Part print with two shaded views. Sizes in mm from the minimum x, y, z corner. A direction names the side the tool comes from. Give positions to 0.01 mm unless a question says otherwise; leave off trailing zeros. Write each loop counter-clockwise with the first axis right and the second up, starting at its lowest first coordinate (ties: lowest second). Pieces come first, ordered by that corner, then holes.
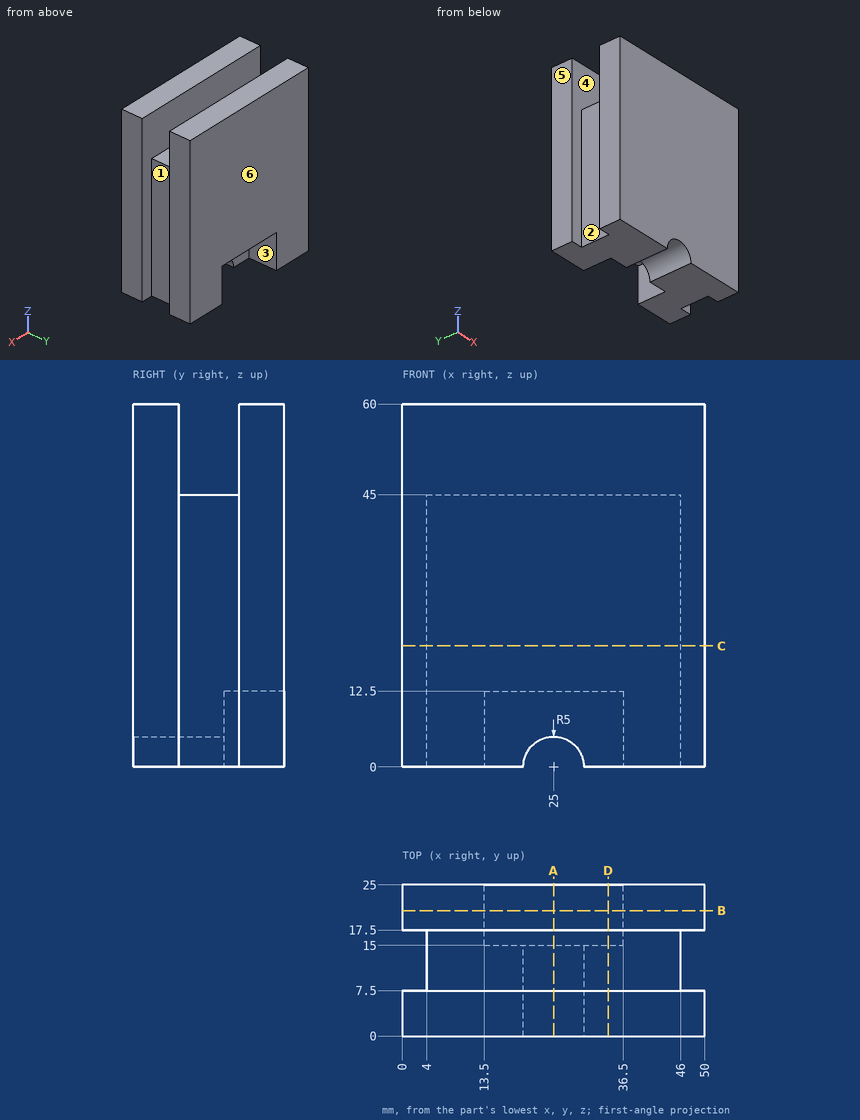
(1) Mould opens along Y. For the marked faces 4, 5 and 6 say: +Y half, -Y half, draft (parallel to the pull), parting line (faces both ways), or undercut.
(2) Saw through at C-C, the plane z = 20. List the corners of the cut face in (x, y).
(3) Saw through at A-A, the plane x = 25. List the corners of the cut face in (y, z).
(4) 3-axis set-ups, long thin cutter, end or side, ignore diameter. For the marked faces 1, 2 and 3: which of +Z, -Z, +X, -X, +Y, -Y reach the whole face in a straight line?
(5) Saw through at D-D, the plane x = 34. List the corners of the cut face in (y, z).
(6) Probe line 1 (Y direction, x = 47, z = 26); line 2 (Z direction, x = 26, y = 22); line 3 (X direction, y = 20.75, z = 11). List the from-to ranges inside material, lowest first.
(7) Drop flat-ended pins along their axis: pin 1 (1.5 mm diameter, centred on x = 35.5, y = 10, fed in from +Z); pin 2 (8 mm diameter, centred on y = 12, z = 19, fed in from -X); pin 3 (14 mm diameter, centred on x = 25, z = 5, fed in from +Y); pin 4 (5 mm diameter, centred on y = 6, z = 50.5, fed in from -X). Give the stop position or say it passes through.
(8) Saw through at B-B, the plane y = 20.75. List the corners of the cut face in (x, z).
Computed values:
1. face 4: undercut
1. face 5: draft
1. face 6: +Y half
2. outline: (0, 0) - (50, 0) - (50, 7.5) - (46, 7.5) - (46, 17.5) - (50, 17.5) - (50, 25) - (0, 25) - (0, 17.5) - (4, 17.5) - (4, 7.5) - (0, 7.5) - close
3. outline: (0, 5) - (15, 5) - (15, 12.5) - (25, 12.5) - (25, 60) - (17.5, 60) - (17.5, 45) - (7.5, 45) - (7.5, 60) - (0, 60) - close
4. face 1: +Z, -Z, +X
4. face 2: +Z, -Z, -X
4. face 3: -Z, +Y
5. outline: (0, 0) - (15, 0) - (15, 12.5) - (25, 12.5) - (25, 60) - (17.5, 60) - (17.5, 45) - (7.5, 45) - (7.5, 60) - (0, 60) - close
6. line 1: y = 0 to 7.5, 17.5 to 25
6. line 2: z = 12.5 to 60
6. line 3: x = 0 to 13.5, 36.5 to 50
7. pin 1: stops at z = 45
7. pin 2: stops at x = 4
7. pin 3: stops at y = 15
7. pin 4: stops at x = 0
8. outline: (0, 0) - (13.5, 0) - (13.5, 12.5) - (36.5, 12.5) - (36.5, 0) - (50, 0) - (50, 60) - (0, 60) - close
